Check sheet for the drawn part. Datum: minimum x, y, z corner. Units: mm. A direction names the side the tool comes from. Round coordinates to 2 decimals unless told otherwise and drop trailing zeros. Write each loop counter-clockwise with the first axis right and the second up, starting at its lowest first coordinate (ties: lowest second). Pieces come first, ordered by that corner, then holes. Notation, with made-up numbers: (72.5, 33) - (79.5, 33) arc R16 ccw to (79.5, 49) - close; hole circle Ø6 at (-37.5, 39.5). An arc over 180 degrees is marked (long way). Answer as a JSON object with one key per item and string values.
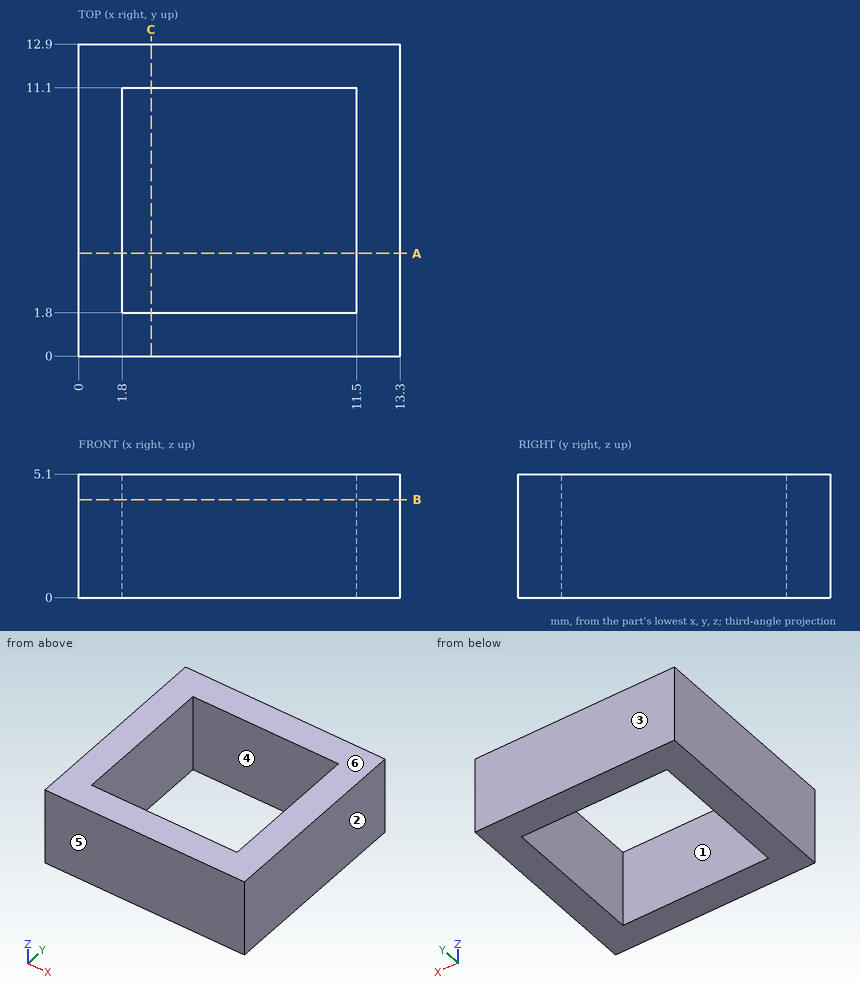
1. Cross-section at A-A (y = 4.25). Record the boundary of the cut face in (x, z).
Completed:
{"outline": "(0, 0) - (1.8, 0) - (1.8, 5.1) - (0, 5.1) - close; (11.5, 0) - (13.3, 0) - (13.3, 5.1) - (11.5, 5.1) - close"}
2. Access from +Z, -Z, +X, -X, +Y, -Y to the whole of each face (thin tool, end or side, straight path). Record for the marked faces 1 and 2.
Completed:
{"face 1": "+Z, -Z", "face 2": "+Z, -Z, +X, +Y, -Y"}
3. Cross-section at C-C (x = 3). Record the boundary of the cut face in (y, z), plus the area to 3 significant figures.
Completed:
{"outline": "(0, 0) - (1.8, 0) - (1.8, 5.1) - (0, 5.1) - close; (11.1, 0) - (12.9, 0) - (12.9, 5.1) - (11.1, 5.1) - close", "area": "18.4 mm^2"}
4. Mould release check, pull along Y, two halves, no side actions. Record for the marked faces 3, 4, 5 and 6: released by +Y, released by -Y, zero draft, split by the parting line, or undercut.
Completed:
{"face 3": "released by +Y", "face 4": "undercut", "face 5": "released by -Y", "face 6": "zero draft"}
5. Go/stop test with a flat-tipped pin: pin 1 (3 mm diameter, centred on x = 4.5, y = 7.5, fed in from +Z). Record where the tip stops, or that it passes through.
Completed:
{"pin 1": "passes through"}
6. Cross-section at B-B (z = 4.05). Record the boundary of the cut face in (x, y), plus the area to 3 significant figures.
Completed:
{"outline": "(0, 0) - (13.3, 0) - (13.3, 12.9) - (0, 12.9) - close; hole (1.8, 1.8) - (11.5, 1.8) - (11.5, 11.1) - (1.8, 11.1) - close", "area": "81.4 mm^2"}
7. Material ranges on probe 1 along Y at (x, z) = (11, 2); probe 2 along X at (y, z) = (3, 4.1), recorded low to high. Write a range as from..to.
Completed:
{"probe 1": "y = 0..1.8, 11.1..12.9", "probe 2": "x = 0..1.8, 11.5..13.3"}
